Here's how the part is built. I have some questions about the finished solid (model axes, mm). A direction names the side the tool comes from. Round coordinates to 2 decimals unless told otherwise and drop trailing zeros. Order: outer loops, then holes, each group sorted by start corner. A loop starts at its lowest first (then second) coordinate and runs counter-clockwise, first axis right, second up. Notation, with made-up numbers: (46.5, 74.25) - (104.5, 74.25) arc R22 cw to (104.5, 81.25) - close; hole circle Ø3 at (52.5, 80). An arc over 180 degrees is marked (long way). One line per item, written item: value.
from build123d import *

# Parameters (mm, degrees)
F0_W      = 12.7
F0_H      = 25.4
F1_DEPTH  = 25.4
F3_DEPTH  = 25.4
F5_DEPTH  = 25.4
F6_W      = 12.7
F6_H      = 12.7
F7_DEPTH  = 12.7
F8_R      = 9.525
F8_R_2    = 6.35
F9_DEPTH  = 12.7
F11_DEPTH = 25.4


with BuildPart() as f1:
    # F0 (on Top) → F1 (new body)
    with BuildSketch(Plane.XY):
        with Locations((-6.35, 0)):
            Rectangle(F0_W, F0_H)
    extrude(amount=F1_DEPTH)

    # F2 (on face) → F3 (cut)
    with BuildSketch(Plane.YZ):
        Polygon((-12.7, 19.05), (-6.35, 25.4), (-12.7, 25.4), align=None)
    extrude(amount=-F3_DEPTH, mode=Mode.SUBTRACT)

    # F4 (on face) → F5 (cut)
    with BuildSketch(Plane.YZ):
        Polygon((12.7, 25.4), (6.35, 25.4), (12.7, 19.05), align=None)
    extrude(amount=-F5_DEPTH, mode=Mode.SUBTRACT)

    # F6 (on face) → F7 (join)
    with BuildSketch(Plane.YZ):
        with Locations((0, 12.7)):
            Rectangle(F6_W, F6_H)
    extrude(amount=F7_DEPTH)


with BuildPart() as f9:
    # F8 (on Front) → F9 (new body, symmetric)
    with BuildSketch(Plane.XZ):
        with Locations((15.9044696867, 12.7)):
            Circle(F8_R)
        with Locations((15.9044696867, 12.7)):
            Circle(F8_R_2, mode=Mode.SUBTRACT)
    extrude(amount=F9_DEPTH, both=True)


with BuildPart() as f1_1:
    add(f1.part)

    # F10: union F9
    add(f9.part)

    # F11 (cut): a face of the model
    f11_faces = [f1_1.faces().sort_by_distance(p)[0] for p in [
        (11.4105492836, -6.35, 12.7),
    ]]
    extrude(f11_faces, amount=-F11_DEPTH, mode=Mode.SUBTRACT)


solid = f1_1.part
Q1. If we section it at D-D, the plane x = -9: Please give me the cut outline in (y, z), then the cut area to 3 significant figures.
Results list:
outline: (-12.7, 0) - (12.7, 0) - (12.7, 19.05) - (6.35, 25.4) - (-6.35, 25.4) - (-12.7, 19.05) - close
area: 605 mm²
Q2. If I drill on line 1 along Z through (x, y) = (16, 5.25); line 2 along X through (y, z) = (7, 13.75); line 3 along Y through (x, z) = (1, 18.75), over which ranges is the centre line in solid material (lowest first)?
Results list:
line 1: 3.18 to 6.35, 19.05 to 22.22
line 2: -12.7 to 0, 6.44 to 9.64, 22.17 to 25.37
line 3: -6.35 to 6.35
Q3. If we section it at C-C, the plane y = -0.5: Please give me the cut outline in (x, z) (3 decimals).
Results list:
outline: (-12.7, 0) - (0, 0) - (0, 6.35) - (8.805, 6.35) arc R9.525 ccw (long way) to (8.805, 19.05) - (0, 19.05) - (0, 25.4) - (-12.7, 25.4) - close; hole circle Ø12.7 at (15.904, 12.7)
Q4. Will these pins go through, and if not, where does the flat tip stop? pin 1 (5 mm diameter, centred on x = -1, y = -5.5, fed in from -Z); pin 2 (2.5 mm diameter, centred on x = 5, z = 12.5, fed in from -Y); pin 3 (4.5 mm diameter, centred on x = 6, y = -1, fed in from -Z); pin 4 (1.5 mm diameter, centred on x = 3.5, y = 0.5, fed in from +Z).
Results list:
pin 1: z = 0
pin 2: y = -6.35
pin 3: z = 6.35
pin 4: z = 19.05
Q5. If we section it at B-B, the plane x = 15: Please give me the cut outline in (y, z), then the cut area to 3 significant figures.
Results list:
outline: (-12.7, 3.22) - (12.7, 3.22) - (12.7, 6.41) - (-12.7, 6.41) - close; (-12.7, 18.99) - (12.7, 18.99) - (12.7, 22.18) - (-12.7, 22.18) - close
area: 162 mm²
Q6. If we section it at A-A, the plane z = 12.7: Please give me the cut outline in (x, y), then the cut area to 3 significant figures.
Results list:
outline: (-12.7, -12.7) - (0, -12.7) - (0, -6.35) - (6.38, -6.35) - (6.38, -12.7) - (9.55, -12.7) - (9.55, 12.7) - (6.38, 12.7) - (6.38, 6.35) - (0, 6.35) - (0, 12.7) - (-12.7, 12.7) - close; (22.25, -12.7) - (25.43, -12.7) - (25.43, 12.7) - (22.25, 12.7) - close
area: 565 mm²
Q7. Which directions (+Z, -Z, +X, -X, +Y, -Y) give clear straight access to the entire face, cutting with the end or side of a thin tool? Please do faces 1 (the flat face through (4, 0, 6.35)), 2 (the flat face through (-6.26, -9.57, 22.18)), 3 (the flat face through (0, 0, 4)), 4 (the flat face through (4, 0, 19.05)), 5 (the flat face through (-6.26, 9.48, 22.27)).
Results list:
face 1: -Z, +Y, -Y
face 2: +Z, -X, -Y
face 3: none
face 4: +Z, +Y, -Y
face 5: +Z, -X, +Y
